Source: CAD feature listing. Evaluate the final solid. Frame: model axes, mm. A direction names the side the tool comes from. Give positions to 0.01 mm unless a question says otherwise; leave off trailing zeros. Order: outer loops, then holes, each group sorted by start corner. A loop starts at its lowest first (then second) coordinate and runs counter-clockwise, first axis right, second up. Notation, with made-up numbers: (-39.5, 76.5) - (-19.5, 76.5) arc R17 cw to (-19.5, 91.5) - close; hole circle Ø9 at (74, 3). An arc over 180 degrees is marked (long way). One line per item, written item: value. Start each with the question number.
from build123d import *

# Parameters (mm, degrees)
SKETCH1_W           = 43
SKETCH1_H           = 37
BOSS_EXTRUDE1_DEPTH = 32
SKETCH2_W           = 10
SKETCH2_H           = 37
CUT_EXTRUDE1_DEPTH  = 25
SKETCH3_R           = 2.5
BOSS_EXTRUDE2_DEPTH = 15


with BuildPart() as part:
    # Sketch1 → Boss-Extrude1 (new body)
    with BuildSketch(Plane.XY):
        with Locations((21.5, -18.5)):
            Rectangle(SKETCH1_W, SKETCH1_H)
    extrude(amount=BOSS_EXTRUDE1_DEPTH)

    # Sketch2 → Cut-Extrude1 (cut)
    with BuildSketch(Plane.XY.offset(32)):
        with Locations((5, -18.5)):
            Rectangle(SKETCH2_W, SKETCH2_H)
    extrude(amount=-CUT_EXTRUDE1_DEPTH, mode=Mode.SUBTRACT)

    # Sketch3 → Boss-Extrude2 (add)
    with BuildSketch(Plane.XY.offset(7)):
        with Locations((5, -6)):
            Circle(SKETCH3_R)
        with Locations((5, -14)):
            Circle(SKETCH3_R)
        with Locations((5, -22)):
            Circle(SKETCH3_R)
        with Locations((5, -30)):
            Circle(SKETCH3_R)
    extrude(amount=BOSS_EXTRUDE2_DEPTH)


solid = part.part
1. Section D-D on y = -23.5. Return the cut outline in (x, z), then the cut area to 3 significant figures.
2. Section A-A on z = 20. Return the cut outline in (x, y).
3. Section C-C on x = 6.5. Return the cut outline in (y, z).
4. Draft query along X for faces 4 (the flat face through (10, -19, 20)), 5 (the flat face through (5, -22, 22)), 6 (the flat face through (0, -19, 3)). Return one class per face: pulls with the +X half, pulls with the -X half, needs draft (parallel to the pull), parting line crosses it, or undercut.
5. Set-up query: faces 1 (the flat face through (43, -19, 16)), 2 (the cylindrical face through (7.385, -5.249, 14.395)), 3 (the flat face through (5, -6, 22)). Return all of +Z, -Z, +X, -X, +Y, -Y with unobstructed straight access to the full face (end or side cutting, diameter ignored); none if empty.
6. Contact query for flat-ended pins moving along their axis: pin 1 Ø2 at (y, z) = (-21, 24) entering from -X; pin 2 Ø1.5 at (y, z) = (-22.5, 19) entering from -X; pin 3 Ø2.5 at (x, y) = (4.5, -29.5) entering from +Z. Output: stop coordinate, or through.
7. Section B-B on y = -14. Return the cut outline in (x, z), then the cut area to 3 significant figures.
8. Ray query, L1, parallel to X at y = -11.5, z = 29.5; L2, parallel to X at y = -23, z = 18.5; L3, parallel to Z at x = 3, y = -25.5. Return the intervals inside material, ascending.
Data:
1. outline: (0, 0) - (43, 0) - (43, 32) - (10, 32) - (10, 7) - (7, 7) - (7, 22) - (3, 22) - (3, 7) - (0, 7) - close
1. area: 1,190 mm2
2. outline: circle Ø5 at (5, -30); circle Ø5 at (5, -22); circle Ø5 at (5, -14); circle Ø5 at (5, -6); (10, -37) - (43, -37) - (43, 0) - (10, 0) - close
3. outline: (-37, 0) - (0, 0) - (0, 7) - (-4, 7) - (-4, 22) - (-8, 22) - (-8, 7) - (-12, 7) - (-12, 22) - (-16, 22) - (-16, 7) - (-20, 7) - (-20, 22) - (-24, 22) - (-24, 7) - (-28, 7) - (-28, 22) - (-32, 22) - (-32, 7) - (-37, 7) - close
4. face 4: undercut
4. face 5: needs draft
4. face 6: pulls with the -X half
5. face 1: +Z, -Z, +X, +Y, -Y
5. face 2: +Z
5. face 3: +Z, -X, +Y, -Y
6. pin 1: stops at x = 10
6. pin 2: stops at x = 2.5
6. pin 3: stops at z = 22
7. outline: (0, 0) - (43, 0) - (43, 32) - (10, 32) - (10, 7) - (7.5, 7) - (7.5, 22) - (2.5, 22) - (2.5, 7) - (0, 7) - close
7. area: 1,200 mm2
8. L1: x = 10 to 43
8. L2: x = 2.71 to 7.29, 10 to 43
8. L3: z = 0 to 7
